The model under review builds one solid part; all positions refer to its coordinate system, in mm. A direction names the side the tool comes from. Round coordinates to 2 decimals unless told otherwise and drop trailing zeros. Order: outer loops, then holes, each group sorted by start corner. A loop starts at its lowest first (then second) coordinate and runs counter-clockwise, first axis right, second up. Notation, with made-up numbers: M -23.5,69 L -16.5,69 A25 ccw -16.5,89 Z; hole C 1.5,-33.75 d7. An arc over 180 degrees is marked long. Answer as a JSON object with one key per item and string values. Group by question number.
1. Mouldability with a two-part tool opening along Z and no side actions: class faces 3 (the face through (2.54, -3.61, -266.58)), 4 (the face through (2.465, -45.302, -232.777)), 5 (the face through (2, 0, -239)) as released by +Z, released by -Z, zero draft, split by the parting line, or undercut.
2. Machinability: for faces 1 (the face through (2, -39, -270)), 2 (the face through (2.54, -0.89, -54.56)), which of the approach directions +Z, -Z, +X, -X, +Y, -Y give a long, thin tool a straight path to every point of the face, cutting with its end or side? Answer none if there is none.
3. Add section D-D on z = -165. State the section outline as (x, y) points, and give its area (3 significant figures).
4. Add section B-B on z = -66. State the section outline as (x, y) points, and give its area (3 significant figures).
5. Clearance check with a flat-ended pin moving along its axis: P1, Ø1.5, axis at x = 0.5, z = -152.5, coming from the +Y side. State where the tip first meets the part, or that it passes through.
6. Add section C-C on x = 2.15. Give the number of separate pieces and of enclosed holes in the cut face, and give its area (3 significant figures).
7. Add section A-A on y = -43.5. State the section outline as (x, z) points, and give its area (3 significant figures).
8. To check wall thickness, follow probe 1 along Y at (x, z) = (3.15, -31.5); probe 2 along Y at (x, z) = (1.1, -38.5); probe 3 along Z at (x, y) = (2.3, -50.5). State the ranges of each line that lie inside material, in increasing order. Write a range as [from, to].
```python
from build123d import *

# Parameters (mm, degrees)
SKETCH1_R           = 6
SKETCH1_R_2         = 2
SKETCH1_R_3         = 1.5
BOSS_EXTRUDE1_DEPTH = 5
FILLET1_R           = 6
FILLET2_R           = 12


with BuildPart() as part:
    # Sketch1 → Boss-Extrude1 (new body)
    with BuildSketch(Plane(origin=(0, 0, 0), x_dir=(0, 0, -1), z_dir=(1, 0, 0))):
        Polygon((0, 0), (55, 0), (75, -20), (195, -20), (215, 0), (270, 0), (270, -72), (0, -72), align=None)
        with Locations((31.5, -43.5)):
            Circle(SKETCH1_R, mode=Mode.SUBTRACT)
        with Locations((55.5, -10)):
            Circle(SKETCH1_R_2, mode=Mode.SUBTRACT)
        with Locations((7.5, -10)):
            Circle(SKETCH1_R_2, mode=Mode.SUBTRACT)
        with Locations((38.5, -59)):
            Circle(SKETCH1_R_3, mode=Mode.SUBTRACT)
        with Locations((25.076606241, -51.25)):
            Circle(SKETCH1_R_3, mode=Mode.SUBTRACT)
        with Locations((25.076606241, -35.75)):
            Circle(SKETCH1_R_3, mode=Mode.SUBTRACT)
        with Locations((38.5, -28)):
            Circle(SKETCH1_R_3, mode=Mode.SUBTRACT)
        with Locations((51.923393759, -35.75)):
            Circle(SKETCH1_R_3, mode=Mode.SUBTRACT)
        with Locations((51.923393759, -51.25)):
            Circle(SKETCH1_R_3, mode=Mode.SUBTRACT)
        with Locations(Location((214.5, -10, 0), (0, 0, 180))):
            Circle(SKETCH1_R_2, mode=Mode.SUBTRACT)
        with Locations(Location((238.5, -9.276470083, 0), (0, 0, 180))):
            Circle(SKETCH1_R_2, mode=Mode.SUBTRACT)
        with Locations(Location((262.5, -10, 0), (0, 0, 180))):
            Circle(SKETCH1_R_2, mode=Mode.SUBTRACT)
        with Locations(Location((244.923393759, -35.75, 0), (0, 0, 180))):
            Circle(SKETCH1_R_3, mode=Mode.SUBTRACT)
        with Locations(Location((231.5, -28, 0), (0, 0, 180))):
            Circle(SKETCH1_R_3, mode=Mode.SUBTRACT)
        with Locations(Location((218.076606241, -35.75, 0), (0, 0, 180))):
            Circle(SKETCH1_R_3, mode=Mode.SUBTRACT)
        with Locations(Location((218.076606241, -51.25, 0), (0, 0, 180))):
            Circle(SKETCH1_R_3, mode=Mode.SUBTRACT)
        with Locations(Location((231.5, -59, 0), (0, 0, 180))):
            Circle(SKETCH1_R_3, mode=Mode.SUBTRACT)
        with Locations(Location((244.923393759, -51.25, 0), (0, 0, 180))):
            Circle(SKETCH1_R_3, mode=Mode.SUBTRACT)
        with Locations(Location((238.5, -43.5, 0), (0, 0, 180))):
            Circle(SKETCH1_R, mode=Mode.SUBTRACT)
        with Locations((31.5, -10)):
            Circle(SKETCH1_R_2, mode=Mode.SUBTRACT)
    extrude(amount=BOSS_EXTRUDE1_DEPTH)

    # Fillet1
    fillet1_edges = [part.edges().sort_by_distance(p)[0] for p in [
        (2.5, -72, -270),
        (2.5, -72, 0),
    ]]
    fillet(fillet1_edges, radius=FILLET1_R)

    # Fillet2
    fillet2_edges = [part.edges().sort_by_distance(p)[0] for p in [
        (2.5, 0, 0),
        (2.5, 0, -55),
        (2.5, -20, -75),
        (2.5, -20, -195),
        (2.5, 0, -215),
        (2.5, 0, -270),
    ]]
    fillet(fillet2_edges, radius=FILLET2_R)


solid = part.part
```
Recorded:
{
 "1": {"face 3": "released by -Z", "face 4": "undercut", "face 5": "zero draft"},
 "2": {"face 1": "-Z, +X, -X, +Y, -Y", "face 2": "+X, -X, +Y"},
 "3": {"outline": "M 0,-72 L 5,-72 L 5,-20 L 0,-20 Z", "area": "260 mm²"},
 "4": {"outline": "M 0,-72 L 5,-72 L 5,-11 L 0,-11 Z", "area": "305 mm²"},
 "5": {"P1": "stops at y = -20"},
 "6": {"separate pieces": "1", "enclosed holes": "20", "area": "16,200 mm²"},
 "7": {"outline": "M 0,-270 L 5,-270 L 5,-244.5 L 0,-244.5 Z; M 0,-232.5 L 5,-232.5 L 5,-37.5 L 0,-37.5 Z; M 0,-25.5 L 5,-25.5 L 5,0 L 0,0 Z", "area": "1,230 mm²"},
 "8": {"probe 1": "y = [-72, -49.5], [-37.5, -12], [-8, 0]", "probe 2": "y = [-72, -60.5], [-57.5, -29.5], [-26.5, 0]", "probe 3": "z = [-270, -246.22], [-243.62, -219.38], [-216.78, -53.22], [-50.62, -26.38], [-23.78, 0]"}
}
